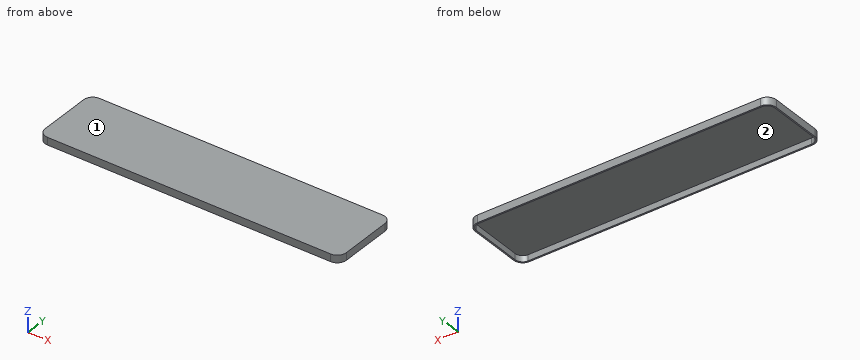
```python
from build123d import *

# Parameters (mm, degrees)
SKETCH002_W    = 202
SKETCH002_H    = 47
PAD001_DEPTH   = 5
FILLET001_R    = 6
THICKNESS001_T = -1


with BuildPart() as part:
    # Sketch002 → Pad001 (new body)
    with BuildSketch(Plane.XY):
        Rectangle(SKETCH002_W, SKETCH002_H)
    extrude(amount=PAD001_DEPTH)

    # Fillet001
    fillet001_edges = [part.edges().sort_by_distance(p)[0] for p in [
        (-101, -23.5, 2.5),
        (101, -23.5, 2.5),
        (-101, 23.5, 2.5),
        (101, 23.5, 2.5),
    ]]
    fillet(fillet001_edges, radius=FILLET001_R)

    # Thickness001
    thickness001_openings = [part.faces().sort_by_distance(p)[0] for p in [
        (0, 0, 0),
    ]]
    offset(amount=THICKNESS001_T, openings=thickness001_openings)


solid = part.part
```
Part model, mm, in its own coordinate system. Face numbers are marked on the shaded views. Coordinates: 2 decimals unless noted, no trailing zeros. Write each loop counter-clockwise with the first axis right and the second up, starting at its lowest first coordinate (ties: lowest second). Pieces come first, ordered by that corner, then holes.
Item 1: Slice it at B-B (y = 6). Write the cut outline in (x, z).
Item 2: Probe line 1 (Y direction, x = -13.5, z = 0.7); line 2 (X direction, y = 3.5, z = 1.1); line 3 (Z direction, x = 77, y = 14). List the from-to ranges inside material, lowest first.
Item 3: Pin check, flat tip, straight feed: pin 1 (5 mm diameter, centred on x = -52.5, y = 17.5, fed in from -Z). Stop position of the tip, or through.
Item 4: Slice it at A-A (z = 2.85). Write the cut outline in (x, y).
Item 5: Slice it at C-C (x = 10.5). Write the cut outline in (y, z), and give its area (3 significant figures).
Item 6: Mould opens along X. For the marked faces 1 and 2 say: released by +X, released by -X, zero draft, split by the parting line, or undercut.
Results found:
1. outline: (-101, 0) - (-100, 0) - (-100, 4) - (100, 4) - (100, 0) - (101, 0) - (101, 5) - (-101, 5) - close
2. line 1: y = -23.5 to -22.5, 22.5 to 23.5
2. line 2: x = -101 to -100, 100 to 101
2. line 3: z = 4 to 5
3. pin 1: stops at z = 4
4. outline: (-101, -17.5) arc R6 ccw to (-95, -23.5) - (95, -23.5) arc R6 ccw to (101, -17.5) - (101, 17.5) arc R6 ccw to (95, 23.5) - (-95, 23.5) arc R6 ccw to (-101, 17.5) - close; hole (-100, -17.5) arc R5 ccw to (-95, -22.5) - (95, -22.5) arc R5 ccw to (100, -17.5) - (100, 17.5) arc R5 ccw to (95, 22.5) - (-95, 22.5) arc R5 ccw to (-100, 17.5) - close
5. outline: (-23.5, 0) - (-22.5, 0) - (-22.5, 4) - (22.5, 4) - (22.5, 0) - (23.5, 0) - (23.5, 5) - (-23.5, 5) - close
5. area: 55.0 mm2
6. face 1: zero draft
6. face 2: undercut
